from build123d import *

# Parameters (mm, degrees)
MAINBODY_DEPTH = 1.5875


with BuildPart() as part:
    # Sketch2 → MainBody (new body)
    with BuildSketch(Plane(origin=(0, -3.4417, 0), x_dir=(-1, 0, 0), z_dir=(0, -1, 0))):
        with BuildLine():
            Line((-50.8, 63.5), (50.8, 63.5))
            ThreePointArc((50.8, 63.5), (59.780256121, 59.780256121), (63.5, 50.8))
            Line((63.5, 50.8), (63.5, -50.8))
            ThreePointArc((63.5, -50.8), (59.780256121, -59.780256121), (50.8, -63.5))
            Line((50.8, -63.5), (-50.8, -63.5))
            ThreePointArc((-50.8, -63.5), (-59.780256121, -59.780256121), (-63.5, -50.8))
            Line((-63.5, -50.8), (-63.5, 50.8))
            ThreePointArc((-63.5, 50.8), (-59.780256121, 59.780256121), (-50.8, 63.5))
        make_face()
        with BuildLine():
            Line((45.992219207, 53.26253), (-45.992219207, 53.26253))
            ThreePointArc((-45.992219207, 53.26253), (-52.726513272, 50.473094065), (-55.515949207, 43.7388))
            Line((-55.515949207, 43.7388), (-55.515949207, -43.7388))
            ThreePointArc((-55.515949207, -43.7388), (-52.726513272, -50.473094065), (-45.992219207, -53.26253))
            Line((-45.992219207, -53.26253), (45.992219207, -53.26253))
            ThreePointArc((45.992219207, -53.26253), (52.726513272, -50.473094065), (55.515949207, -43.7388))
            Line((55.515949207, -43.7388), (55.515949207, 0))
            Line((55.515949207, 0), (55.515949207, 43.7388))
            ThreePointArc((55.515949207, 43.7388), (52.726513272, 50.473094065), (45.992219207, 53.26253))
        make_face(mode=Mode.SUBTRACT)
    extrude(amount=MAINBODY_DEPTH)


solid = part.part
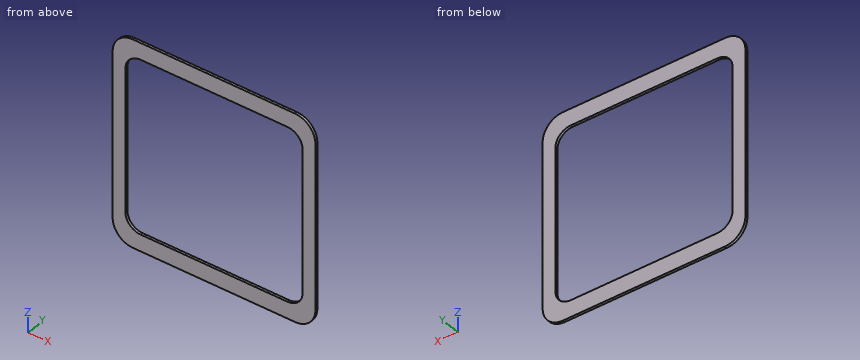
Design review of the part built by this model. Coordinates are the model's own, in mm. Coordinates: 2 decimals unless noted, no trailing zeros. Loops run counter-clockwise (first coordinate to the right, second up) from the corner with the lowest first, then second, coordinate; pieces in that order, holes last.
Item 1: Wall thickness on L1, parallel to Z at x = -36, y = -3.85; L2, parallel to X at y = -4.9, z = -33; L3, parallel to Z at x = 58, y = -4.4: over which ranges is each line inside the solid? List them lowest first.
Completed:
L1: z = -63.5 to -53.26, 53.26 to 63.5
L2: x = -63.5 to -55.52, 55.52 to 63.5
L3: z = -61.26 to 61.26
Item 2: Add section A-A (z = -33). Write out the cut boundary in (x, y).
Completed:
outline: (-63.5, -5.03) - (-55.52, -5.03) - (-55.52, -3.44) - (-63.5, -3.44) - close; (55.52, -5.03) - (63.5, -5.03) - (63.5, -3.44) - (55.52, -3.44) - close
Item 3: Add section B-B (x = 34). Write out the cut boundary in (y, z), and give its area (3 significant figures).
Completed:
outline: (-5.03, -63.5) - (-3.44, -63.5) - (-3.44, -53.26) - (-5.03, -53.26) - close; (-5.03, 53.26) - (-3.44, 53.26) - (-3.44, 63.5) - (-5.03, 63.5) - close
area: 32.5 mm2
Item 4: Add section C-C (y = -3.85). Write out the cut boundary in (x, z).
Completed:
outline: (-63.5, -50.8) arc R12.7 ccw to (-50.8, -63.5) - (50.8, -63.5) arc R12.7 ccw to (63.5, -50.8) - (63.5, 50.8) arc R12.7 ccw to (50.8, 63.5) - (-50.8, 63.5) arc R12.7 ccw to (-63.5, 50.8) - close; hole (-55.52, -43.74) arc R9.52 ccw to (-45.99, -53.26) - (45.99, -53.26) arc R9.52 ccw to (55.52, -43.74) - (55.52, 43.74) arc R9.52 ccw to (45.99, 53.26) - (-45.99, 53.26) arc R9.52 ccw to (-55.52, 43.74) - close
